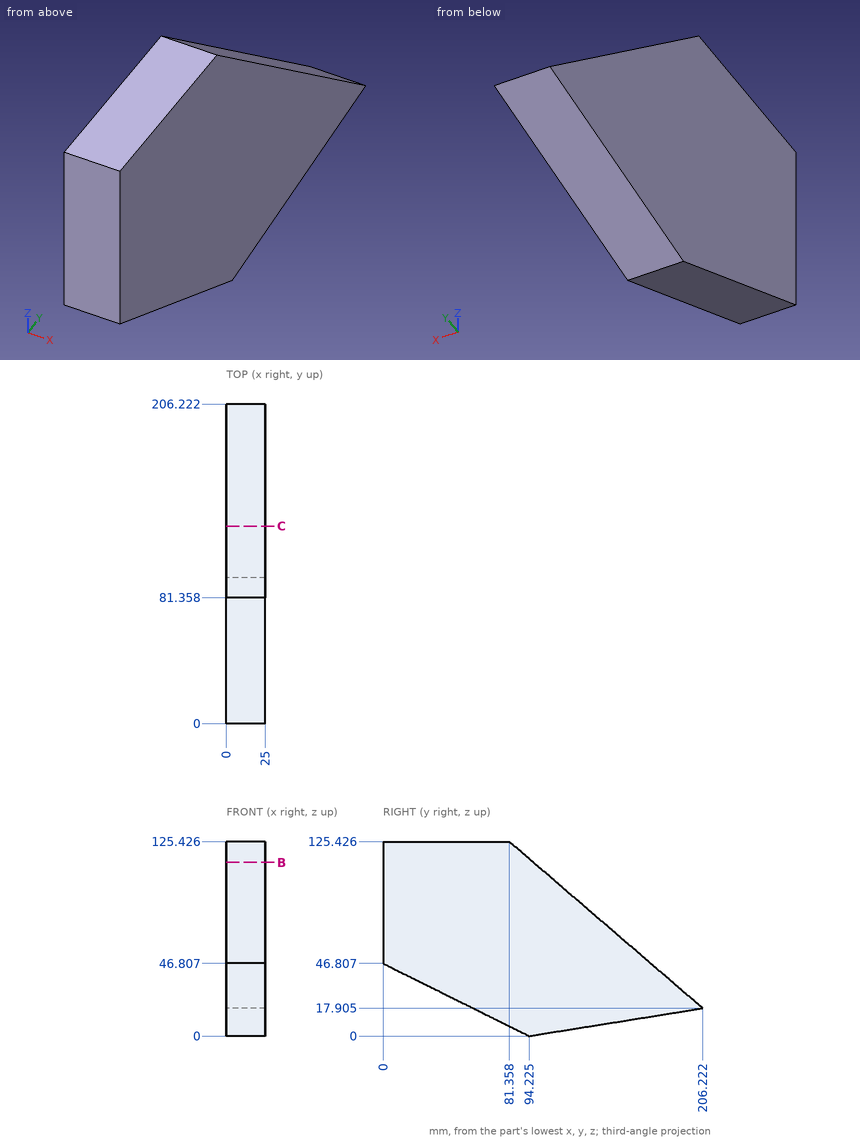
Part print with two shaded views. Sizes in mm from the minimum x, y, z corner. Round coordinates to 2 decimals unless told otherwise and drop trailing zeros. Loops run counter-clockwise (first coordinate to the right, second up) from the corner with the lowest first, then second, coordinate; pieces in that order, holes last.
1. Drill centre lines: line 1 along Z through (x, y) = (22.5, 87); line 2 along Y through (x, z) = (23, 31.5) (1 decimal); line 3 along Z through (x, y) = (11, 126) (1 decimal). Where is each one in solid material? Low to high.
Solutions:
line 1: z = 3.59 to 120.57
line 2: y = 30.8 to 190.4
line 3: z = 5.1 to 87
2. Slice it at C-C (y = 127.5). Give the cut face in (x, z).
Solutions:
outline: (0, 5.32) - (25, 5.32) - (25, 85.69) - (0, 85.69) - close
3. Flat gauge pins, fed straight in: pin 1 (10 mm diameter, centred on x = 8.5, y = 185, fed in from -Z); pin 2 (12 mm diameter, centred on x = 5, z = 79.5, fed in from -Y); pin 3 (4 mm diameter, centred on x = 3.5, z = 16, fed in from +Y); pin 4 (1.5 mm diameter, centred on x = 6.5, z = 26.5, fed in from +Y). Where does each tip first touch, or does it go through?
Solutions:
pin 1: stops at z = 13.71
pin 2: stops at y = 0
pin 3: stops at y = 206.22
pin 4: stops at y = 197.11
4. Slice it at B-B (z = 112). Give the cut face in (x, y).
Solutions:
outline: (0, 0) - (25, 0) - (25, 96.95) - (0, 96.95) - close
